from build123d import *

# Parameters (mm, degrees)
CORTE_EXTRUS_O1_REACH = 208
ESBO_O2_R             = 2.5
ESBO_O4_R             = 2.5
CORTE_EXTRUS_O2_DEPTH = 50
ESBO_O5_R             = 2.5
CORTE_EXTRUS_O3_DEPTH = 110


with BuildPart() as part:
    # Esboço1 → Revolução1 (revolve)
    with BuildSketch(Plane.XY, mode=Mode.PRIVATE) as revolu_o1_sk:
        with BuildLine():
            Line((0, 0), (10, 0))
            Line((10, 0), (34.5, 10.652173913))
            Line((34.5, 10.652173913), (34.5, 86.956521739))
            Line((34.5, 86.956521739), (37.5, 86.956521739))
            Line((37.5, 86.956521739), (37.5, 11.956521739))
            Line((37.5, 11.956521739), (59.250106277, 21.413089686))
            ThreePointArc((59.250106277, 21.413089686), (64.360493758, 26.432550668), (64.802782332, 33.582056216))
            Line((64.802782332, 33.582056216), (12.5, 200))
            Line((12.5, 200), (0, 200))
            Line((0, 200), (0, 203))
            Line((0, 203), (14.701817656, 203))
            Line((14.701817656, 203), (67.664763483, 34.481536006))
            ThreePointArc((67.664763483, 34.481536006), (67.089788336, 25.187178794), (60.446284612, 18.661879517))
            Line((60.446284612, 18.661879517), (37.5, 8.685234034))
            Line((37.5, 8.685234034), (37.5, -3))
            Line((37.5, -3), (10.623961722, -3))
            Line((10.623961722, -3), (0, -3))
            Line((0, -3), (0, 0))
        make_face()
    revolve(revolu_o1_sk.sketch.rotate(Axis((0, 0, 0), (0, 1, 0)), 90), axis=Axis((0, 0, 0), (0, 1, 0)))  # turned: the seam where the file's is

    # Esboço2 → Corte-extrusão1 (cut, up to next)
    with BuildSketch(Plane.XZ.offset(3), mode=Mode.PRIVATE) as corte_extrus_o1_sk1:
        with Locations(Location((0, 0, 0), (0, 0, 270))):  # turned: the seam where the file's is
            Circle(ESBO_O2_R)
    corte_extrus_o1_tool1 = extrude(corte_extrus_o1_sk1.sketch, amount=-CORTE_EXTRUS_O1_REACH, mode=Mode.PRIVATE) & part.part
    add(corte_extrus_o1_tool1.solids().sort_by_distance((0, -3, 0))[0], mode=Mode.SUBTRACT)

    # Esboço4 → Corte-extrusão2 (cut)
    with BuildSketch(Plane(origin=(0, 0, 0), x_dir=(0, 0, -1), z_dir=(1, 0, 0))):
        with Locations(Location((0, 162.819249831, 0), (0, 0, 306.470564915))):  # turned: the seam where the file's is
            Circle(ESBO_O4_R)
    extrude(amount=CORTE_EXTRUS_O2_DEPTH, mode=Mode.SUBTRACT)

    # Esboço5 → Corte-extrusão3 (cut)
    with BuildSketch(Plane.XY):
        with Locations(Location((0, 57.186880689, 0), (0, 0, 90))):  # turned: the seam where the file's is
            Circle(ESBO_O5_R)
    extrude(amount=-CORTE_EXTRUS_O3_DEPTH, mode=Mode.SUBTRACT)


solid = part.part
Work out the finished part from the listing and answer in its coordinate system (mm). A direction names the side the tool comes from. Give positions to 0.01 mm unless a question says otherwise; leave off trailing zeros. Loops run counter-clockwise (first coordinate to the right, second up) from the corner with the lowest first, then second, coordinate; pieces in that order, holes last. Notation, with made-up numbers: (84.5, -22.5) - (122.5, -22.5) arc R24 cw to (122.5, 12.5) - close; hole circle Ø5 at (-10.75, 13.5). An arc over 180 degrees is marked (long way). Answer in a Markdown table with one row per item. Add a question column.
Q1. Consider line 1 along X through (y, z) = (78, -29); line 2 along X through (y, z) = (-2.4, 0); line 3 along Z through (x, y) = (1, 24). Determine where each line is inside the solid, lowest interval first.
Q2. The part is cut by section A-A (y = 50.5). Determine the outline of the cut face in (x, z), and give its area (4 significant figures).
Q3. The part is cut by section D-D (y = 143). Determine the outline of the cut face in (x, z).
Q4. A tool of negligible diameter and unlimited length cuts with its end or side. For faces 1 (the cylindrical face through (33.27, 2.76, -17.3)), 2 (the conical face through (-11.434, 0.666, 1.501)), 3 (the cylindrical face through (0.958, 59.496, -58.923)), from which of +Z, -Z, +X, -X, +Y, -Y can it reach the whole face along a straight path? Write none if from no direction.
Q5. Each of these flat-tipped pins is pushed along its axis until it touches: P1, Ø1, axis at x = 31, z = -48, coming from the -Y side; P2, Ø4, axis at x = 0, y = 57.19, coming from the +Z side; P3, Ø8, axis at y = 35, z = -38.5, coming from the +X side. Where does it stop, or does it pass through?
Q6. The part is cut by section C-C (x = 0). State how many separate pieces and enclosed holes the cut face has, and give its area (3 significant figures).
Q7. The part is cut by section B-B (y = 93). Determine the outline of the cut face in (x, z).
Q8. Determine the mould class of faces 4 (the conical face through (-11.67, 12.55, -37.07)), 5 (the conical face through (34.26, 9.17, -17.82)), 6 (the flat face through (8, -3, 1)) for opening direction X: released by +X, released by -X, zero draft, split by the parting line, or undercut.
Solution:
| question | item | result |
|---|---|---|
| 1 | line 1 | x = -45.54 to -41.76, -23.77 to -18.69, 18.69 to 23.77, 41.76 to 45.54 |
| 1 | line 2 | x = -37.5 to -2.5, 2.5 to 37.5 |
| 1 | line 3 | z = -66.46 to -62.78, -37.49 to -34.49, 34.49 to 37.49, 62.78 to 66.46 |
| 2 | outline | circle Ø125.26 at (0, 0); circle Ø75 at (0, 0); hole circle Ø118.97 at (0, 0); hole circle Ø69 at (0, 0) |
| 2 | area | 1,885 mm² |
| 3 | outline | circle Ø67.12 at (0, 0); hole circle Ø60.83 at (0, 0) |
| 4 | face 1 | -Y |
| 4 | face 2 | none |
| 4 | face 3 | -Z |
| 5 | P1 | stops at y = 17.01 |
| 5 | P2 | stops at z = 61.16 |
| 5 | P3 | stops at x = 58.35 |
| 6 | separate pieces | 3 |
| 6 | enclosed holes | 0 |
| 6 | area | 2,340 mm² |
| 7 | outline | circle Ø98.55 at (0, 0); hole circle Ø92.26 at (0, 0) |
| 8 | face 4 | undercut |
| 8 | face 5 | split by the parting line |
| 8 | face 6 | zero draft |
